Autodesk Inventor part; units mm, degrees
ref_plane "YZ Plane" through (0, 0, 0) normal (1, 0, 0) x (0, 1, 0)
ref_plane "XZ Plane" through (0, 0, 0) normal (0, 1, 0) x (-1, 0, 0)
ref_plane "XY Plane" through (0, 0, 0) normal (0, 0, 1) x (1, 0, 0)
sketch "Sketch1" plane through (0, 0, 0) normal (0, 0, 1) x (1, 0, 0)
  circle A0 centre (30, 26.4525) radius 3
  circle A1 centre (-30, 26.4525) radius 3
  line L0 (-12, 6.73) -> (12, 6.73)
  line L1 (12, 6.73) -> (12, 13)
  line L2 (12, 13) -> (-12, 13)
  line L3 (-12, 13) -> (-12, 6.73)
  line L4 (0, 33.0213) -> (0, 0)
  circle A2 centre (30, 26.4525) radius 3.05
  circle A3 centre (-30, 26.4525) radius 3.05
  line L5 (37.7199, 32.4525) -> (0, 32.4525)
  line L6 (0, 32.4525) -> (0, 20.4525)
  line L7 (0, 20.4525) -> (37.7199, 20.4525)
  line L8 (37.7199, 20.4525) -> (37.7199, 32.4525)
  circle A4 centre (30, 26.4525) radius 6 construction
  dimension "d0" = 6.1
  dimension "d1" = 6.1
  dimension "d12" = 3
extrude "Extrusion1" add sketch "Sketch1" against normal blind 10 contours L4 L5 L8 L7
sketch "Sketch2" plane through (0, 0, 0) normal (0, 0, 1) x (1, 0, 0)
  circle A0 centre (30, 26.4525) radius 3.05
  line L0 (0, 20.4525) -> (0, 32.4525)
  circle A1 centre (0, 26.4525) radius 2.45
  circle A2 centre (14.0354, 26.4525) radius 2.45
  dimension "d13" = 4.9
  dimension "d14" = 4.9
extrude "Extrusion2" cut sketch "Sketch2" against normal blind 4 contours A1 L0 | L0 A1 | A2
sketch "Sketch3" plane through (37.7199, 20.4525, 0) normal (1, 0, 0) x (0, 0, -1)
  line L0 (0, 0) -> (0, 12)
  line L1 (0, 0) -> (10, 0)
  line L2 (10, 12) -> (10, 0)
  line L3 (0, 12) -> (10, 12)
  circle A0 centre (5, 6) radius 1.45
  point P0 (0, -20.4525)
  dimension "d15" = 2.9
extrude "Extrusion3" cut sketch "Sketch3" against normal up to surface contours A0
ref_plane "Work Plane1" through (37.7199, 32.4525, 0) normal (0.7071, 0.7071, 0) x (0, 0, 1)
mirror "Mirror2" about plane through (0, 20.4525, 0) normal (-1, 0, 0) of "Extrusion1", "Extrusion2", "Extrusion3"
sketch "Sketch5" plane through (0, 0, 0) normal (0, 0, 1) x (1, 0, 0)
  point P0 (0, 0)
sketch "Sketch6" plane through (0, 0, 0) normal (0, 0, 1) x (1, 0, 0)
  circle A0 centre (-14.0354, 26.4525) radius 2.45
  circle A1 centre (-14.0354, 26.4525) radius 4.05
  point P0 (0, 0)
  dimension "d31" = 8.1
extrude "Extrusion5" cut sketch "Sketch6" against normal blind 3 contours A0 | A1
ref_plane "Work Plane2" through (-37.7199, 32.4525, 0) normal (0.7071, -0.7071, 0) x (0, 0, 1)
properties part number "cellSTORM_inverted_sampleholder_bar"
Input: part model. Units: mm. Frame: model coordinates. A direction names the side the tool comes from. Coordinates: 2 decimals unless noted, no trailing zeros. Write each loop counter-clockwise with the first axis right and the second up, starting at its lowest first coordinate (ties: lowest second). Pieces come first, ordered by that corner, then holes. Notation, with made-up numbers: (12, -24.5) -> (53, -24.5) arc R22 ccw to (53, 10.5) -> close; hole circle Ø9 at (35, 67). An arc over 180 degrees is marked (long way). Answer as a JSON object with one key per item and string values.
1. Access query for faces 1 (the face through (-12.23, 24.797, -3.493)), 2 (the face through (-35.24, 26.39, -3.55)), 3 (the face through (-1, 29, 0)), 4 (the face through (-1, 20.452, -5)), 5 (the face through (35.24, 26.52, -3.55)). Directions: +Z, -Z, +X, -X, +Y, -Y. A direction counts if a zero-diameter tool reaches every point of the face in a straight line with its end or side. Return the directions, or none.
Result set:
{"face 1": "+Z", "face 2": "-X", "face 3": "+Z, +X, -X, +Y, -Y", "face 4": "+Z, -Z, +X, -X, -Y", "face 5": "+X"}
2. Section C-C on x = 0. Return the cut outline in (y, z), then the cut area to 3 significant figures.
Result set:
{"outline": "(20.45, -10) -> (32.45, -10) -> (32.45, 0) -> (28.9, 0) -> (28.9, -4) -> (24, -4) -> (24, 0) -> (20.45, 0) -> close", "area": "100 mm2"}
3. First-contact query: P1, Ø2.5, axis at x = 0.5, y = 25.5, coming from the +Z side; P2, Ø2.5, axis at x = -15, y = 24.5, coming from the +Z side. Flat tips, straight axial feed; report the tip coordinate or a pass-through.
Result set:
{"P1": "stops at z = -4", "P2": "stops at z = -3"}
4. Section A-A on x = -30. Return the cut outline in (y, z).
Result set:
{"outline": "(20.45, -10) -> (23.4, -10) -> (23.4, 0) -> (20.45, 0) -> close; (29.5, -10) -> (32.45, -10) -> (32.45, 0) -> (29.5, 0) -> close"}
5. Material intervals for line 1 (X direction, y = 27, z = -3.5); line 2 (Y direction, x = -34.75, z = -5); line 3 (X direction, y = 24.5, z = -4.25), sorted ascending. Write a range as from..to.
Result set:
{"line 1": "x = -37.72..-33, -27..-16.42, -11.65..-2.39, 2.39..11.65, 16.42..27, 33..37.72", "line 2": "y = 20.45..25, 27.9..32.45", "line 3": "x = -37.72..-32.34, -27.66..27.66, 32.34..37.72"}
6. Section D-D on y = 25.75. Count the separate pieces of the cut face and the enclosed holes in it, then the cut area to 3 significant figures.
Result set:
{"separate pieces": "5", "enclosed holes": "0", "area": "545 mm2"}
7. Section B-B on z = -5. Return the cut outline in (x, y).
Result set:
{"outline": "(-37.72, 20.45) -> (37.72, 20.45) -> (37.72, 25) -> (32.68, 25) arc R3.05 cw (long way) to (32.68, 27.9) -> (37.72, 27.9) -> (37.72, 32.45) -> (-37.72, 32.45) -> (-37.72, 27.9) -> (-32.68, 27.9) arc R3.05 cw (long way) to (-32.68, 25) -> (-37.72, 25) -> close"}
8. Mould query, pull axis X, two halves, no side actions, for faces 6 (the face through (-37.72, 25, -4)), 7 (the face through (1, 32.452, -5)), 8 (the face through (0.319, 24.023, -1.972)). Classes: released by +X, released by -X, zero draft, split by the parting line, or undercut.
Result set:
{"face 6": "released by -X", "face 7": "zero draft", "face 8": "undercut"}
